Build history of the part. All positions in model axes, mm. Face numbers are marked on the shaded views. Round coordinates to 2 decimals unless told otherwise and drop trailing zeros. Write each loop counter-clockwise with the first axis right and the second up, starting at its lowest first coordinate (ties: lowest second). Pieces come first, ordered by that corner, then holes. Notation, with made-up numbers: (-31, 60.5) -> (27, 60.5) arc R30 cw to (27, 87.5) -> close; hole circle Ø7 at (21.5, -1.5). An arc over 180 degrees is marked (long way). Return JSON: item names as keys, results as strings.
Autodesk Fusion 360 part; units mm, degrees
sketch "Sketch1" plane through (0, 0, 0) normal (0, 0, 1) x (1, 0, 0)
  line L0 (-7.62, 3.81) -> (-7.62, -3.81)
  line L1 (-3.81, -7.62) -> (3.81, -7.62)
  line L2 (7.62, -3.81) -> (7.62, 3.81)
  line L3 (3.81, 7.62) -> (-3.81, 7.62)
  line L4 (-7.62, 7.62) -> (7.62, -7.62) construction
  line L5 (7.62, 7.62) -> (-7.62, -7.62) construction
  circle A0 centre (0, 0) radius 2.54
  arc A1 (-3.81, 7.62) -> (-7.62, 3.81) centre (-3.81, 3.81) ccw
  arc A2 (-7.62, -3.81) -> (-3.81, -7.62) centre (-3.81, -3.81) ccw
  arc A3 (7.62, 3.81) -> (3.81, 7.62) centre (3.81, 3.81) ccw
  arc A4 (3.81, -7.62) -> (7.62, -3.81) centre (3.81, -3.81) ccw
  dimension "d1" = 5.08
  dimension "d2" = 3.81
  dimension "d3" = 7.62
  dimension "d5" = 3.81
  dimension "d6" = 3.81
  dimension "d7" = 3.81
extrude "Extrude1" add sketch "Sketch1" against normal blind 50.8
sketch "Sketch2" plane through (0, 7.62, 0) normal (0, 1, 0) x (-1, 0, 0)
  line L0 (3.81, 0) -> (-3.81, 0)
  line L1 (3.81, -50.8) -> (3.81, 0)
  line L2 (-3.81, -50.8) -> (3.81, -50.8)
  line L3 (-3.81, 0) -> (-3.81, -50.8)
  circle A0 centre (0, 0) radius 0.9525
  dimension "d11" = 1.905
extrude "Extrude2" cut sketch "Sketch2" against normal through all contours L0 A0 picked at (0.2327, 0.216)
sketch "Sketch3" plane through (-7.62, 0, 0) normal (-1, 0, 0) x (0, 0, 1)
  line L0 (0, -3.81) -> (0, 3.81)
  line L1 (-50.8, -3.81) -> (0, -3.81)
  line L2 (-50.8, 3.81) -> (-50.8, -3.81)
  line L3 (0, 3.81) -> (-50.8, 3.81)
  circle A0 centre (0, 0) radius 0.9525
  dimension "d13" = 1.905
extrude "Extrude3" cut sketch "Sketch3" against normal through all contours L0 A0 picked at (0.2079, 0.24)
equation "d2 = d3 / 2"
equation "d3 = d1 / 2 + WireInsulationLength"
equation "WireInsulationLength = 0.2 in"
equation "d5 = d3 / 2"
equation "d6 = d3 / 2"
equation "d7 = d3 / 2"
equation "d8 = -2\""
equation "WireChannelDiameter = 0.075 in"
equation "d11 = WireChannelDiameter"
equation "d13 = WireChannelDiameter"
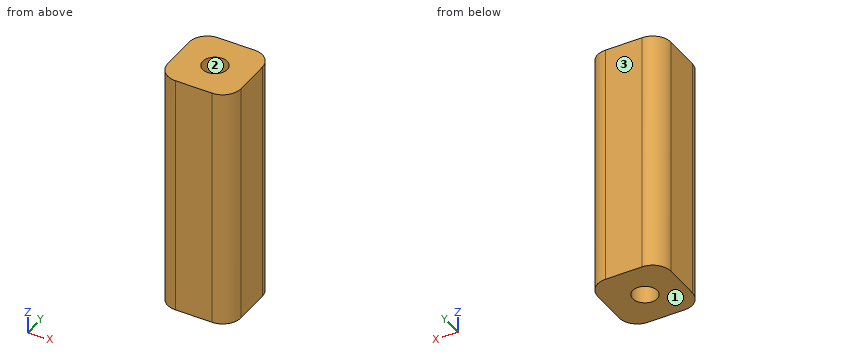
Q1. Two-plate mould, pull along Y, no slides. Class the marked faces 1, 2 and 3: +Y half, -Y half, draft (parallel to the pull), parting line (faces both ways), or undercut.
Verdict:
{"face 1": "draft", "face 2": "undercut", "face 3": "+Y half"}
Q2. Wall check: L1, parallel to X at y = 0, z = -28; L2, parallel to Y at x = -2, z = -39. Give the ranges that are in metal, low to high.
Verdict:
{"L1": "x = -7.62 to -2.54, 2.54 to 7.62", "L2": "y = -7.62 to -1.57, 1.57 to 7.62"}
Q3. Saw through at C-C on z = -21.5. List the corners of the cut face in (x, y).
Verdict:
{"outline": "(-7.62, -3.81) arc R3.81 ccw to (-3.81, -7.62) -> (3.81, -7.62) arc R3.81 ccw to (7.62, -3.81) -> (7.62, 3.81) arc R3.81 ccw to (3.81, 7.62) -> (-3.81, 7.62) arc R3.81 ccw to (-7.62, 3.81) -> close; hole circle Ø5.08 at (0, 0)"}
Q4. Pin check, flat tip, straight feed: pin 1 Ø8 at (x, z) = (-4.5, -42) entering from -Y. Stop position of the tip, or through.
Verdict:
{"pin 1": "stops at y = -7.62"}
Q5. Saw through at A-A on x = 0. List the corners of the cut face in (y, z).
Verdict:
{"outline": "(-7.62, -50.8) -> (-2.54, -50.8) -> (-2.54, 0) -> (-7.62, 0) -> close; (2.54, -50.8) -> (7.62, -50.8) -> (7.62, 0) -> (2.54, 0) -> close"}
Q6. Saw through at D-D on x = 6.25. List the corners of the cut face in (y, z), then the cut area to 3 significant figures.
Verdict:
{"outline": "(-6.74, -50.8) -> (6.74, -50.8) -> (6.74, 0) -> (-6.74, 0) -> close", "area": "684 mm²"}
